```python
from build123d import *

# Parameters (mm, degrees)
F1_DEPTH        = 4
F2_R            = 5
F3_R            = 2
F5_DEPTH        = 6
F6_R            = 5
F8_DEPTH        = 3
F10_F1_R        = 5
F10_F2_R        = 5
F10_2_T1_DEPTH  = 11.6034789136
F10_2_T3_DEPTH  = 16.5
F10_2_T5_DEPTH  = 13.1244047484
F10_2_T8_ANGLE  = 72.2553283749
F10_2_T10_ANGLE = 90


# Not quite as in the source:
# - a fillet or chamfer that OpenCascade refuses, or shapes differently, is made with other operations: its cross-section is extruded or revolved along the edge and cut away or added
# - a pattern or mirror of a feature is missing from the dataset's text; its kind, count and spacing are read off the source's solid


with BuildPart() as f1:
    # F0 (on Top) → F1 (new body)
    with BuildSketch(Plane.XY):
        Polygon((0, 25), (0, 0), (0, -25), (12, -25), (20, 0), (20, 25), align=None)
    extrude(amount=F1_DEPTH)

    # F1_copies: F1 across plane


with BuildPart() as f1_1:
    add(f1.part)
    add(f1.part.mirror(Plane(origin=(0, 0, 0), x_dir=(0, 0, -1), z_dir=(-1, 0, 0))))

    # F2
    f2_edges = [f1_1.edges().sort_by_distance(p)[0] for p in [
        (12, -25, 2),
        (20, 25, 2),
    ]]
    fillet(f2_edges, radius=F2_R)

    # F3
    f3_edges = [f1_1.edges().sort_by_distance(p)[0] for p in [
        (-1.824881, -25, 4),
        (20, 10, 4),
        (11.29817, -24.038527, 4),
        (-16, -12.5, 4),
        (16.556179, -10.761939, 4),
        (-20, 12.5, 4),
        (-2.5, 25, 4),
        (18.535534, 23.535534, 4),
    ]]
    fillet(f3_edges, radius=F3_R)

    # F4 (on Top) → F5 (join)
    with BuildSketch(Plane.XY):
        Polygon((0, 18), (0, 0), (0, -15), (6, -15), (10, 0), (10, 18), align=None)
    f5 = extrude(amount=F5_DEPTH)

    # F5_copies: F5 across plane
    add(f5.mirror(Plane(origin=(0, 0, 0), x_dir=(0, 0, -1), z_dir=(-1, 0, 0))))

    # F6
    f6_edges = [f1_1.edges().sort_by_distance(p)[0] for p in [
        (6, -15, 5),
    ]]
    fillet(f6_edges, radius=F6_R)

    # F10#2: fillet of radius 5 on 3 edges, made by hand

    # F10_2_s2 → F10_2_t1 (cut)
    with BuildSketch(Plane.XY.offset(4)):
        with BuildLine():
            ThreePointArc((-2.1586084346, -15), (-5.2047891364, -13.9649442785), (-6.9897831326, -11.2883132528))
            Line((-6.9897831326, -11.2883132528), (-6, -15))
            Line((-6, -15), (-2.1586084346, -15))
        make_face()
    extrude(amount=F10_2_T1_DEPTH, mode=Mode.SUBTRACT)

    # F10_2_s4 → F10_2_t3 (cut)
    with BuildSketch(Plane.XY.offset(-12.5)):
        with BuildLine():
            ThreePointArc((-15, 25), (-18.5355339059, 23.5355339059), (-20, 20))
            Line((-20, 20), (-20, 25))
            Line((-20, 25), (-15, 25))
        make_face()
    extrude(amount=F10_2_T3_DEPTH, mode=Mode.SUBTRACT)

    # F10_2_s6 → F10_2_t5 (cut)
    with BuildSketch(Plane.XY.offset(-9.1244047484)):
        with BuildLine():
            ThreePointArc((-13.1123588366, -21.5238786355), (-11.2981701574, -24.0385265368), (-8.3502381006, -25))
            Line((-8.3502381006, -25), (-12, -25))
            Line((-12, -25), (-13.1123588366, -21.5238786355))
        make_face()
    extrude(amount=F10_2_T5_DEPTH, mode=Mode.SUBTRACT)

    # F10_2_s7 → F10_2_t8 (revolve, cut)
    with BuildSketch(Plane(origin=(5.0298762867, -15.718363396, 0), x_dir=(0, 0, 1), z_dir=(-0.3047757271, 0.9524241472, 0))):
        with BuildLine():
            ThreePointArc((4, -17.048482944), (3.4142135624, -18.4626965064), (2, -19.048482944))
            Line((2, -19.048482944), (4, -19.048482944))
            Line((4, -19.048482944), (4, -17.048482944))
        make_face()
    revolve(axis=Axis((-8.3502381006, -20, 4), (0, 0, 1)), revolution_arc=F10_2_T8_ANGLE, mode=Mode.SUBTRACT)

    # F10_2_s9 → F10_2_t10 (revolve, cut)
    with BuildSketch(Plane.YZ.offset(-15)):
        with BuildLine():
            ThreePointArc((23, 4), (24.4142135624, 3.4142135624), (25, 2))
            Line((25, 2), (25, 4))
            Line((25, 4), (23, 4))
        make_face()
    revolve(axis=Axis((-15, 20, 4), (0, 0, 1)), revolution_arc=F10_2_T10_ANGLE, mode=Mode.SUBTRACT)



with BuildPart() as f8:
    # F7 (on Top) → F8 (new body)
    with BuildSketch(Plane.XY):
        Polygon((0, 20), (0, 0), (0, -18), (7, -18), (12, 0), (12, 20), align=None)
    extrude(amount=F8_DEPTH)


with BuildPart() as f8_1:
    # F9: moved
    add(f8.part.moved(Location((0, 0, 6))))

    # F10: fillet of radius 5 on 2 edges, made by hand

    # F10_f1
    f10_f1_edges = [f8_1.edges().sort_by_distance(p)[0] for p in [
        (12, 20, 7.5),
    ]]
    fillet(f10_f1_edges, radius=F10_F1_R)

    # F10_f2
    f10_f2_edges = [f8_1.edges().sort_by_distance(p)[0] for p in [
        (7, -18, 7.5),
    ]]
    fillet(f10_f2_edges, radius=F10_F2_R)


with BuildPart() as f1_2:
    add(f1_1.part)

    add(f8_1.part)  # F11 merges F8
    # F11: F8 across plane
    add(f8_1.part.mirror(Plane.YZ))


solid = f1_2.part
```
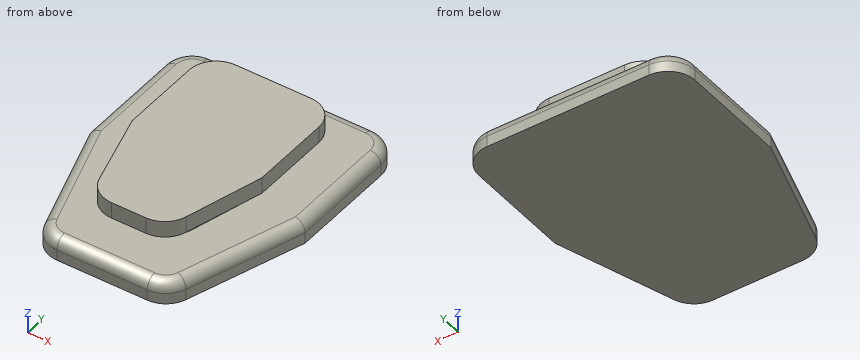
Input: part model. Units: mm. Frame: model coordinates. Give positions to 0.01 mm unless a question says otherwise; leave off trailing zeros. Order: outer loops, then holes, each group sorted by start corner. A loop starts at its lowest first (then second) coordinate and runs counter-clockwise, first axis right, second up. Notation, with made-up numbers: (21, 64) - (58, 64) arc R26 ccw to (58, 85) - close; hole circle Ø5 at (82, 33.5). An arc over 180 degrees is marked (long way). Put each result on its own line as item: value.
Item 1: Ray query, L1, parallel to Z at x = 2, y = -18.5; L2, parallel to X at y = 10.5, z = 5.5; L3, parallel to Y at x = -3.5, z = 6.75. Return the intervals inside material, ascending. Write a range as from..to.
Found:
L1: z = 0..4
L2: x = -10..10
L3: y = -17.99..20
Item 2: Section query A-A, the plane z = 7. Return loops of the section in (x, y), then the cut area to 3 significant figures.
Found:
outline: (-12, 0) - (-8.02, -14.34) arc R5 ccw to (-3.2, -18) - (3.2, -18) arc R5 ccw to (8.02, -14.34) - (12, 0) - (12, 15) arc R5 ccw to (7, 20) - (-7, 20) arc R5 ccw to (-12, 15) - close
area: 806 mm^2
Item 3: Contact query for flat-ended pins moving along their axis: pin 1 (1.5 mm diameter, centred on x = 3.5, z = 8, fed in from +Y); pin 2 (0.9 mm diameter, centred on x = 0.5, z = 7.5, fed in from -Y); pin 3 (1 mm diameter, centred on y = -17.5, z = 3, fed in from -X). Output: stop coordinate, or through.
Found:
pin 1: stops at y = 20
pin 2: stops at y = -18
pin 3: stops at x = -14.4
Item 4: Section query B-B, the plane z = 3. Return loops of the section in (x, y).
Found:
outline: (-19.73, 0.04) - (-12.86, -21.44) arc R4.73 ccw to (-8.35, -24.73) - (8.35, -24.73) arc R4.73 ccw to (12.86, -21.44) - (19.73, 0.04) - (19.73, 20) arc R4.73 ccw to (15, 24.73) - (-15, 24.73) arc R4.73 ccw to (-19.73, 20) - close
